Input: part model. Units: mm. Frame: model coordinates. A direction names the side the tool comes from. Round coordinates to 2 decimals unless told otherwise and drop trailing zeros. Order: outer loops, then holes, each group sorted by start corner. A loop starts at its lowest first (then second) coordinate and runs counter-clockwise, first axis right, second up. Notation, with made-up numbers: (9, 55.25) -> (45, 55.25) arc R33 cw to (45, 85.25) -> close; hole circle Ø6 at (64.25, 70). An arc over 180 degrees is marked (long way). Use a Markdown table: item, result.
from build123d import *

# Parameters (mm, degrees)
SKETCH1_R           = 17.5
SKETCH1_R_2         = 12
BOSS_EXTRUDE1_DEPTH = 26.5
SKETCH2_R           = 12
SKETCH2_R_2         = 6
BOSS_EXTRUDE2_DEPTH = 1
SKETCH3_R           = 14.5
SKETCH3_R_2         = 12
BOSS_EXTRUDE3_DEPTH = 5


with BuildPart() as part:
    # Sketch1 → Boss-Extrude1 (new body)
    with BuildSketch(Plane(origin=(0, 0, 0), x_dir=(1, 0, 0), z_dir=(0, 1, 0))):
        Circle(SKETCH1_R)
        Circle(SKETCH1_R_2, mode=Mode.SUBTRACT)
    extrude(amount=BOSS_EXTRUDE1_DEPTH)

    # Sketch2 → Boss-Extrude2 (add)
    with BuildSketch(Plane(origin=(0, 26.5, 0), x_dir=(1, 0, 0), z_dir=(0, 1, 0))):
        Circle(SKETCH2_R)
        Circle(SKETCH2_R_2, mode=Mode.SUBTRACT)
    extrude(amount=-BOSS_EXTRUDE2_DEPTH)

    # Sketch3 → Boss-Extrude3 (add)
    with BuildSketch(Plane.XZ):
        Circle(SKETCH3_R)
        Circle(SKETCH3_R_2, mode=Mode.SUBTRACT)
    extrude(amount=BOSS_EXTRUDE3_DEPTH)


solid = part.part
1) Contact query for flat-ended pins moving along their axis: P1, Ø8, axis at y = 5.5, z = -0.5, coming from the -X side; P2, Ø1.5, axis at x = 6, y = 11.5, coming from the +Z side; P3, Ø3, axis at y = 12.5, z = -2.5, coming from the +X side; P4, Ø12, axis at y = 15.5, z = 9, coming from the -X side. Output: stop coordinate, or through.
Answer key:
| item | result |
|---|---|
| P1 | stops at x = -17.5 |
| P2 | stops at z = 16.69 |
| P3 | stops at x = 17.47 |
| P4 | stops at x = -17.24 |
2) Set-up query: faces 4 (the face through (-6, 26, 0)), 5 (the face through (-7, 0, -13)). Return all of +Z, -Z, +X, -X, +Y, -Y with unobstructed straight access to the full face (end or side cutting, diameter ignored); none if empty.
Answer key:
| item | result |
|---|---|
| face 4 | +Y, -Y |
| face 5 | -Y |
3) Draft query along Z for faces 1 (the face through (-11.99, 10.46, 0.53)), 2 (the face through (6.691, -2.465, -12.864)), 3 (the face through (2, -5, 12)). Return one class per face: released by +Z, released by -Z, zero draft, split by the parting line, or undercut.
Answer key:
| item | result |
|---|---|
| face 1 | undercut |
| face 2 | split by the parting line |
| face 3 | zero draft |
4) Cut plane C-C on y = -3. Return loops of the section in (x, z), and give its area (3 significant figures).
Answer key:
| item | result |
|---|---|
| outline | circle Ø29 at (0, 0); hole circle Ø24 at (0, 0) |
| area | 208 mm^2 |
5) Cut plane D-D on z = 13. Return loops of the section in (x, y), and give its area (3 significant figures).
Answer key:
| item | result |
|---|---|
| outline | (-11.72, 0) -> (-6.42, 0) -> (-6.42, -5) -> (6.42, -5) -> (6.42, 0) -> (11.72, 0) -> (11.72, 26.5) -> (-11.72, 26.5) -> close |
| area | 685 mm^2 |
6) Ray query, probe 1 along Z at (x, y) = (0, 26.25); probe 2 along Z at (x, y) = (0, 19.5). Return the intervals inside material, ascending.
Answer key:
| item | result |
|---|---|
| probe 1 | z = -17.5 to -6, 6 to 17.5 |
| probe 2 | z = -17.5 to -12, 12 to 17.5 |
7) Cut plane A-A on z = 0. Return loops of the section in (x, y).
Answer key:
| item | result |
|---|---|
| outline | (-17.5, 0) -> (-14.5, 0) -> (-14.5, -5) -> (-12, -5) -> (-12, 25.5) -> (-6, 25.5) -> (-6, 26.5) -> (-17.5, 26.5) -> close; (6, 25.5) -> (12, 25.5) -> (12, -5) -> (14.5, -5) -> (14.5, 0) -> (17.5, 0) -> (17.5, 26.5) -> (6, 26.5) -> close |
8) Cut plane B-B on x = 0. Return loops of the section in (y, z).
Answer key:
| item | result |
|---|---|
| outline | (-5, -14.5) -> (0, -14.5) -> (0, -17.5) -> (26.5, -17.5) -> (26.5, -6) -> (25.5, -6) -> (25.5, -12) -> (-5, -12) -> close; (-5, 12) -> (25.5, 12) -> (25.5, 6) -> (26.5, 6) -> (26.5, 17.5) -> (0, 17.5) -> (0, 14.5) -> (-5, 14.5) -> close |
